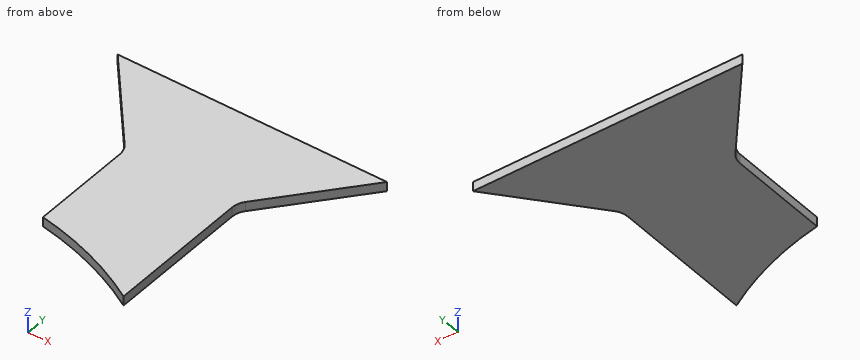
from build123d import *

# Parameters (mm, degrees)
FUNNEL_SIDE_PANEL_DEPTH = 5
FILLET1_R               = 10


with BuildPart() as part:
    # Sketch1 → Funnel - Side Panel (new body)
    with BuildSketch(Plane.XY):
        with BuildLine():
            Line((30, 0), (30, 80))
            Line((30, 80), (71.974030913, 130.022702136))
            Line((71.974030913, 130.022702136), (-71.974030913, 130.022702136))
            Line((-71.974030913, 130.022702136), (-30, 80))
            Line((-30, 80), (-30, 22.326086298))
            ThreePointArc((-30, 22.326086298), (1.02961193, 13.930062634), (30, 0))
        make_face()
    extrude(amount=FUNNEL_SIDE_PANEL_DEPTH)

    # Fillet1
    fillet1_edges = [part.edges().sort_by_distance(p)[0] for p in [
        (-30, 80, 2.5),
        (30, 80, 2.5),
    ]]
    fillet(fillet1_edges, radius=FILLET1_R)


solid = part.part
Source: CAD feature listing. Evaluate the final solid. Frame: model axes, mm. Round coordinates to 2 decimals unless told otherwise and drop trailing zeros. Loops run counter-clockwise (first coordinate to the right, second up) from the corner with the lowest first, then second, coordinate; pieces in that order, holes last. Notation, with made-up numbers: M -37.75,81 L 7.25,81 A14 ccw 7.25,100 Z; hole C 33.25,58 d3. An arc over 180 degrees is marked long. Return JSON: item names as keys, results as strings. Group by question number.
1. Material intervals for line 1 along X through (y, z) = (26, 4.2); line 2 along Y through (x, z) = (-38.5, 1); line 3 along Y through (x, z) = (-3.5, 4), sorted ascending. Write a range as from..to.
2. Pin query (flat end, axial travel): pin 1 (1.5 mm diameter, centred on y = 35.5, z = 3.5, fed in from +X); pin 2 (2 mm diameter, centred on y = 44, z = 3.5, fed in from -X). Return the tip coordinate at first contact, or that it passes through.
3. Section query B-B on y = 16.5. Output: boundary loops of the cut face in (x, z), and give its area (3 significant figures).
4. Section query A-A on z = 2.05. Output: boundary loops of the cut face in (x, y).
5. Section query C-C on x = 23. Output: boundary loops of the cut face in (y, z), and give its area (3 significant figures).
Checks:
{
 "1": {"line 1": "x = -30..30", "line 2": "y = 90.13..130.02", "line 3": "y = 15.55..130.02"},
 "2": {"pin 1": "stops at x = 30", "pin 2": "stops at x = -30"},
 "3": {"outline": "M -6.38,0 L 30,0 L 30,5 L -6.38,5 Z", "area": "182 mm²"},
 "4": {"outline": "M -71.97,130.02 L -32.34,82.79 A10 cw -30,76.36 L -30,22.33 A175 cw 30,0 L 30,76.36 A10 cw 32.34,82.79 L 71.97,130.02 Z"},
 "5": {"outline": "M 3.98,0 L 130.02,0 L 130.02,5 L 3.98,5 Z", "area": "630 mm²"}
}
